Work out the finished part from the listing and answer in its coordinate system (mm). A direction names the side the tool comes from. Give positions to 0.01 mm unless a question says otherwise; leave off trailing zeros. Loops run counter-clockwise (first coordinate to the right, second up) from the corner with the lowest first, then second, coordinate; pieces in that order, holes last. Notation, with made-up numbers: (36, -27) - (42, -27) arc R20 cw to (42, -9) - close; hole circle Ø1 at (54, -12.5). An arc over 180 degrees is marked (long way). One line per question, with ' | ' between items. Start each with the question number.
1. Section C-C (y = 16) is taken. Determine the outline of the cut face in (x, z).
2. Section A-A (z = 35) is taken. Determine the outline of the cut face in (x, y), plus the area to 3 significant figures.
3. Find the intervals of material crossed by line 1 (X direction, y = 1.3, z = -35); line 2 (X direction, y = 6.5, z = 0.5); line 3 (Y direction, x = 37, z = -24), in increasing order.
4. Section D-D (x = 0) is taken. Determine the outline of the cut face in (y, z), plus the area to 3 significant figures.
5. For a pull along Z with two mould halves and no side action, classify faces 6 (the face through (-36.9, 1.5, -36.2)), 7 (the face through (0, 9, -36.164)), 8 (the face through (0, 15, 33)), 9 (the face through (35.1, 1.5, -36.2)) as released by +Z, released by -Z, zero draft, split by the parting line, or undercut.
6. Each of these flat-tipped pins is pushed along its axis until it touches: pin 1 (2.5 mm diameter, centred on y = 8.5, z = -34, fed in from -X); pin 2 (3.5 mm diameter, centred on x = 0, y = 7.5, fed in from -Z); pin 3 (5 mm diameter, centred on y = 16.5, z = 24.5, fed in from -X). Where does it stop, or does it pass through?
7. Which of the six approach directions +Z, -Z, +X, -X, +Y, -Y give full straight-line access (tool end or side, diameter ignored) to faces 1 (the face through (0, 9, -28.063)), 2 (the face through (-7.754, 9, -32)), 3 (the face through (-15, 12, 0)), 4 (the face through (-16, 9, 34)), 5 (the face through (33, 12, 0))?
8. Section B-B (x = -36) is taken. Determine the outline of the cut face in (y, z).
from build123d import *

# Parameters (mm, degrees)
SKETCH1_W           = 84
SKETCH1_H           = 81
BOSS_EXTRUDE1_DEPTH = 3
SKETCH2_W           = 18
SKETCH2_H           = 48
BOSS_EXTRUDE2_DEPTH = 19
SKETCH3_W           = 32
SKETCH3_H           = 20
SKETCH3_W_2         = 15.507070526
SKETCH3_H_2         = 8.100708483
BOSS_EXTRUDE3_DEPTH = 12
SKETCH4_R           = 1.5
CUT_EXTRUDE1_DEPTH  = 12


with BuildPart() as part:
    # Sketch1 → Boss-Extrude1 (new body)
    with BuildSketch(Plane(origin=(0, 0, 0), x_dir=(1, 0, 0), z_dir=(0, 1, 0))):
        Rectangle(SKETCH1_W, SKETCH1_H)
    extrude(amount=BOSS_EXTRUDE1_DEPTH)

    # Sketch2 → Boss-Extrude2 (add)
    with BuildSketch(Plane(origin=(0, 3, 0), x_dir=(1, 0, 0), z_dir=(0, 1, 0))):
        with Locations((-24, 0)):
            Rectangle(SKETCH2_W, SKETCH2_H)
        with Locations((24, 0)):
            Rectangle(SKETCH2_W, SKETCH2_H)
    extrude(amount=BOSS_EXTRUDE2_DEPTH)

    # Sketch3 → Boss-Extrude3 (add)
    with BuildSketch(Plane(origin=(0, 3, 0), x_dir=(1, 0, 0), z_dir=(0, 1, 0))):
        with Locations((0, -33.5)):
            Rectangle(SKETCH3_W, SKETCH3_H)
        with Locations((0, 32.113522915)):
            Rectangle(SKETCH3_W_2, SKETCH3_H_2)
    extrude(amount=BOSS_EXTRUDE3_DEPTH)

    # Sketch4 → Cut-Extrude1 (cut)
    with BuildSketch(Plane(origin=(0, 3, 0), x_dir=(1, 0, 0), z_dir=(0, 1, 0))):
        with Locations(Location((-36, 35, 0), (0, 0, 270))):
            Circle(SKETCH4_R)
        with Locations(Location((36, 35, 0), (0, 0, 270))):
            Circle(SKETCH4_R)
        with Locations(Location((36, -35, 0), (0, 0, 270))):
            Circle(SKETCH4_R)
        with Locations(Location((-36, -35, 0), (0, 0, 270))):
            Circle(SKETCH4_R)
    extrude(amount=-CUT_EXTRUDE1_DEPTH, mode=Mode.SUBTRACT)


solid = part.part
Conclusion:
1) outline: (-33, -24) - (-15, -24) - (-15, 24) - (-33, 24) - close; (15, -24) - (33, -24) - (33, 24) - (15, 24) - close
2) outline: (-42, 0) - (-37.5, 0) - (-37.5, 3) - (-42, 3) - close; (-34.5, 0) - (34.5, 0) - (34.5, 3) - (16, 3) - (16, 15) - (-16, 15) - (-16, 3) - (-34.5, 3) - close; (37.5, 0) - (42, 0) - (42, 3) - (37.5, 3) - close | area: 618 mm²
3) line 1: -42 to -37.5, -34.5 to 34.5, 37.5 to 42 | line 2: -33 to -15, 15 to 33 | line 3: 0 to 3
4) outline: (0, -40.5) - (3, -40.5) - (3, -36.16) - (15, -36.16) - (15, -28.06) - (3, -28.06) - (3, 23.5) - (15, 23.5) - (15, 43.5) - (3, 43.5) - (3, 40.5) - (0, 40.5) - close | area: 580 mm²
5) face 6: undercut | face 7: released by -Z | face 8: zero draft | face 9: undercut
6) pin 1: x = -7.75 | pin 2: z = -36.16 | pin 3: x = -33
7) face 1: +X, -X, +Y | face 2: -Z, -X, +Y | face 3: -Z, +Y | face 4: +Z, -X, +Y | face 5: +Z, -Z, +X, +Y
8) outline: (0, -40.5) - (3, -40.5) - (3, -36.5) - (0, -36.5) - close; (0, -33.5) - (3, -33.5) - (3, 33.5) - (0, 33.5) - close; (0, 36.5) - (3, 36.5) - (3, 40.5) - (0, 40.5) - close
